Here's how the part is built. I have some questions about the finished solid (model axes, mm). A direction names the side the tool comes from. Give positions to 0.01 mm unless a question says otherwise; leave off trailing zeros. Loops run counter-clockwise (first coordinate to the right, second up) from the corner with the lowest first, then second, coordinate; pieces in that order, holes last.
Q1. Will these pins go through, and if not, where does the flat tip stop? P1, Ø7.5, axis at y = 29.5, z = 6, coming from the -X side; P2, Ø2, axis at y = 52.5, z = 45, coming from the +X side; P3, Ø4, axis at y = -3.5, z = 41.5, coming from the -X side.
Q2. If we section it at B-B (y = 63): Please give me the cut outline in (x, z).
Q3. If we section it at A-A (x = 43): Please give me the cut outline in (y, z), plus the area to 3 significant figures.
Q4. If we section it at D-D (y = -7.5): Please give me the cut outline in (x, z), plus the area to 3 significant figures.
Q5. I need wall thicknesses on line 1 (X direction, y = 53, z = 2); line 2 (Y direction, x = 32, z = 9); line 3 (Y direction, x = 24.5, z = 30.5). Which ranges of each line are inside material? Lowest first, please.
Q6. For faces 1 (the face through (55.224, 51, 24)), 2 (the face through (-57, -64.477, 27)), 3 (the face through (-72.646, -53, 35)), which set-ups out of +Z, -Z, +X, -X, +Y, -Y let a thin tool reach every point of the face, with its end or its side?
Q7. We'd pull the mould along Y, two halves only. Please class faces 4 (the face through (-76.27, -46.7, 23.8)), 5 (the face through (68, 41.289, 24)), 6 (the face through (22, -59.837, 24)), 7 (the face through (-63, 18, 0)): +Y half, -Y half, draft (parallel to the pull), parting line (faces both ways), or undercut.
Q8. If we section it at C-C (z = 4.5): Please give me the cut outline in (x, y), plus the area to 3 significant figures.
from build123d import *

# Parameters (mm, degrees)
F1_DEPTH = 48.2772234827
F2_R     = 17.3254122278
F3_DEPTH = 178.0532356352
F6_DEPTH = 147.4594417959
F8_DEPTH = 137.5391036272


with BuildPart() as f1:
    # F0 (on Top) → F1 (new body)
    with BuildSketch(Plane.XY):
        with BuildLine():
            Line((61.5742132068, 73.062568903), (-67.3387721181, 73.062568903))
            Line((-67.3387721181, 73.062568903), (-67.3387721181, 14.0218225376))
            ThreePointArc((-67.3387721181, 14.0218225376), (-81.6301408592, -50.1107967732), (-16.6482494662, -59.8365291953))
            Line((-16.6482494662, -59.8365291953), (61.5742132068, -59.8365291953))
            Line((61.5742132068, -59.8365291953), (61.5742132068, -48.7425401807))
            Line((61.5742132068, -48.7425401807), (74.8133137822, -48.7425401807))
            Line((74.8133137822, -48.7425401807), (74.8133137822, 41.2890613079))
            Line((74.8133137822, 41.2890613079), (61.5742132068, 41.2890613079))
            Line((61.5742132068, 41.2890613079), (61.5742132068, 73.062568903))
        make_face()
        with BuildLine():
            Line((-60.9887721181, 66.712568903), (55.2242132068, 66.712568903))
            Line((55.2242132068, 66.712568903), (55.2242132068, 34.9390613079))
            Line((55.2242132068, 34.9390613079), (68.4633137822, 34.9390613079))
            Line((68.4633137822, 34.9390613079), (68.4633137822, -42.3925401807))
            Line((68.4633137822, -42.3925401807), (55.2242132068, -42.3925401807))
            Line((55.2242132068, -42.3925401807), (55.2242132068, -53.4865291953))
            Line((55.2242132068, -53.4865291953), (-18.9623394024, -53.4865291953))
            ThreePointArc((-18.9623394024, -53.4865291953), (-76.785621878, -45.9365465001), (-60.9887721181, 10.1971668335))
            Line((-60.9887721181, 10.1971668335), (-60.9887721181, 66.712568903))
        make_face(mode=Mode.SUBTRACT)
    extrude(amount=F1_DEPTH)

    # F2 (on face) → F3 (cut)
    with BuildSketch(Plane(origin=(0, 73.062568903, 0), x_dir=(-1, 0, 0), z_dir=(0, 1, 0))):
        with Locations((19.0455075353, 25.0077471137)):
            Circle(F2_R)
    extrude(amount=-F3_DEPTH, mode=Mode.SUBTRACT)

    # F5 (on face) → F6 (cut)
    with BuildSketch(Plane.YZ.offset(74.8133137822)):
        with BuildLine():
            Line((-48.7425401807, 17.1086588609), (-48.7425401807, 44.9944263589))
            ThreePointArc((-48.7425401807, 44.9944263589), (-56.7710567622, 31.0515426099), (-48.7425401807, 17.1086588609))
        make_face()
        with BuildLine():
            ThreePointArc((-48.7425401807, 17.1086588609), (-32.6051243829, 17.0807615663), (-24.5283525081, 31.0515426099))
            ThreePointArc((-24.5283525081, 31.0515426099), (-32.6051243829, 45.0223236536), (-48.7425401807, 44.9944263589))
            Line((-48.7425401807, 44.9944263589), (-48.7425401807, 17.1086588609))
        make_face()
    extrude(amount=-F6_DEPTH, mode=Mode.SUBTRACT)

    # F7 (on face) → F8 (cut)
    with BuildSketch(Plane(origin=(0, 73.062568903, 0), x_dir=(-1, 0, 0), z_dir=(0, 1, 0))):
        with BuildLine():
            ThreePointArc((67.3387721181, 15.4306932509), (71.3607365337, 20.4974204611), (72.7954935712, 26.8053039908))
            ThreePointArc((72.7954935712, 26.8053039908), (71.3607365337, 33.1131875206), (67.3387721181, 38.1799147308))
            Line((67.3387721181, 38.1799147308), (67.3387721181, 15.4306932509))
        make_face()
        with BuildLine():
            Line((67.3387721181, 15.4306932509), (67.3387721181, 38.1799147308))
            ThreePointArc((67.3387721181, 38.1799147308), (43.6282399612, 26.8053039908), (67.3387721181, 15.4306932509))
        make_face()
    extrude(amount=-F8_DEPTH, mode=Mode.SUBTRACT)


solid = f1.part
Check sheet entries:
1. P1: stops at x = -67.34
1. P2: stops at x = 61.57
1. P3: stops at x = -85.2
2. outline: (-67.34, 0) - (-60.99, 0) - (-60.99, 12.49) arc R14.58 cw to (-67.34, 15.43) - close; (-67.34, 38.18) arc R14.58 cw to (-60.99, 41.12) - (-60.99, 48.28) - (-67.34, 48.28) - close; (55.22, 0) - (61.57, 0) - (61.57, 48.28) - (55.22, 48.28) - close
3. outline: (-59.84, 0) - (-53.49, 0) - (-53.49, 21.3) arc R16.12 cw to (-53.49, 40.8) - (-53.49, 48.28) - (-59.84, 48.28) - close; (66.71, 0) - (73.06, 0) - (73.06, 48.28) - (66.71, 48.28) - close
3. area: 569 mm2
4. outline: (-86.08, 0) - (-79.11, 0) - (-79.11, 48.28) - (-86.08, 48.28) - close; (68.46, 0) - (74.81, 0) - (74.81, 48.28) - (68.46, 48.28) - close
4. area: 643 mm2
5. line 1: x = -67.34 to -60.99, 55.22 to 61.57
5. line 2: y = -59.84 to -53.49, 66.71 to 73.06
5. line 3: y = -59.84 to -56.76, 66.71 to 73.06
6. face 1: +Z, -Z
6. face 2: +Y
6. face 3: +X
7. face 4: undercut
7. face 5: +Y half
7. face 6: -Y half
7. face 7: draft
8. outline: (-67.34, 14.02) arc R44.9 ccw (long way) to (-16.65, -59.84) - (61.57, -59.84) - (61.57, -48.74) - (74.81, -48.74) - (74.81, 41.29) - (61.57, 41.29) - (61.57, 73.06) - (-67.34, 73.06) - close; hole (-60.99, 10.2) arc R38.55 ccw (long way) to (-18.96, -53.49) - (55.22, -53.49) - (55.22, -42.39) - (68.46, -42.39) - (68.46, 34.94) - (55.22, 34.94) - (55.22, 66.71) - (-60.99, 66.71) - close
8. area: 3,490 mm2
